```python
from build123d import *

# Parameters (mm, degrees)
ESQUISSE1_W             = 255
ESQUISSE1_H             = 150
BOSS_EXTRU_1_DEPTH      = 10
ENL_V_MAT_EXTRU_1_DEPTH = 10


with BuildPart() as part:
    # Esquisse1 → Boss.-Extru.1 (new body)
    with BuildSketch(Plane.XY):
        Rectangle(ESQUISSE1_W, ESQUISSE1_H)
    extrude(amount=BOSS_EXTRU_1_DEPTH)

    # Esquisse2 → Enlèv. mat.-Extru.1 (cut)
    with BuildSketch(Plane(origin=(0, 0, 0), x_dir=(-1, 0, 0), z_dir=(0, 0, -1))):
        Polygon((-89.5, 75), (-89.5, 65), (-91.05, 65), (-91.05, 59.5), (-89.5, 59.5), (-89.5, 53.5), (-85.5, 53.5), (-85.5, 59.5), (-83.95, 59.5), (-83.95, 65), (-85.5, 65), (-85.5, 75), align=None)
        Polygon((0.5, 75), (0.5, 65), (-1.05, 65), (-1.05, 59.5), (0.5, 59.5), (0.5, 53.5), (4.5, 53.5), (4.5, 59.5), (6.05, 59.5), (6.05, 65), (4.5, 65), (4.5, 75), align=None)
        Polygon((90.5, 75), (90.5, 65), (88.95, 65), (88.95, 59.5), (90.5, 59.5), (90.5, 53.5), (94.5, 53.5), (94.5, 59.5), (96.05, 59.5), (96.05, 65), (94.5, 65), (94.5, 75), align=None)
        Polygon((94.5, -75), (94.5, -65), (96.05, -65), (96.05, -59.5), (94.5, -59.5), (94.5, -53.5), (90.5, -53.5), (90.5, -59.5), (88.95, -59.5), (88.95, -65), (90.5, -65), (90.5, -75), align=None)
        Polygon((4.5, -75), (4.5, -65), (6.05, -65), (6.05, -59.5), (4.5, -59.5), (4.5, -53.5), (0.5, -53.5), (0.5, -59.5), (-1.05, -59.5), (-1.05, -65), (0.5, -65), (0.5, -75), align=None)
        Polygon((-85.5, -75), (-85.5, -65), (-83.95, -65), (-83.95, -59.5), (-85.5, -59.5), (-85.5, -53.5), (-89.5, -53.5), (-89.5, -59.5), (-91.05, -59.5), (-91.05, -65), (-89.5, -65), (-89.5, -75), align=None)
    extrude(amount=-ENL_V_MAT_EXTRU_1_DEPTH, mode=Mode.SUBTRACT)


solid = part.part
```
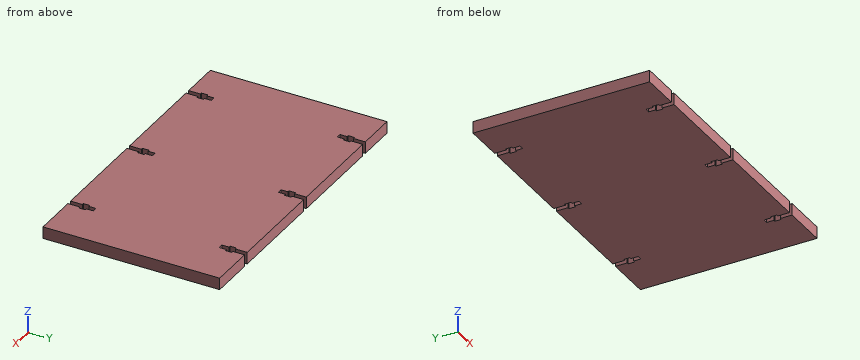
CAD build for the part. Positions are in the model's coordinates, mm. Give positions to 0.01 mm unless a question says otherwise; leave off trailing zeros. Write each loop counter-clockwise with the first axis right and the second up, starting at its lowest first coordinate (ties: lowest second). Pieces come first, ordered by that corner, then holes. Notation, with made-up numbers: M 22.25,-13.75 L 50.25,-13.75 A13 ccw 50.25,2.25 Z; hole C -25,-36.75 d10. An arc over 180 degrees is marked long. Return JSON: item names as keys, results as strings. Group by question number.
(1) Flat gauge pin, fed straight in: pin 1 Ø1.2 at (x, z) = (-3, 3.5) entering from +Y. Where does the tip first touch, or does it go through?
(2) Drill centre lines: L1, parallel to X at y = 63.5, z = 4.75; L2, parallel to X at y = 67, z = 4.25; L3, parallel to Y at x = -2, z = 3. Where is each one in solid material? Low to high. Write a range as [from, to].
(3) Band-saw the part on A-A (y = -62.5). Give the cut face in (x, z).
Entries:
{
 "1": {"pin 1": "stops at y = 53.5"},
 "2": {"L1": "x = [-127.5, -96.05], [-88.95, -6.05], [1.05, 83.95], [91.05, 127.5]", "L2": "x = [-127.5, -94.5], [-90.5, -4.5], [-0.5, 85.5], [89.5, 127.5]", "L3": "y = [-53.5, 53.5]"},
 "3": {"outline": "M -127.5,0 L -96.05,0 L -96.05,10 L -127.5,10 Z; M -88.95,0 L -6.05,0 L -6.05,10 L -88.95,10 Z; M 1.05,0 L 83.95,0 L 83.95,10 L 1.05,10 Z; M 91.05,0 L 127.5,0 L 127.5,10 L 91.05,10 Z"}
}
